For this review, take the finished solid that the model builds, in its own axes (mm). A direction names the side the tool comes from. Round coordinates to 2 decimals unless told otherwise and drop trailing zeros. Write each loop counter-clockwise with the first axis right and the second up, starting at its lowest first coordinate (ties: lowest second). Pieces come first, ordered by that corner, then holes.
from build123d import *

# Parameters (mm, degrees)
F1_DEPTH  = 43
F2_R      = 4
F3_DEPTH  = 6
F4_R      = 1.5
F5_DEPTH  = 25
F4_R_2    = 3
F6_DEPTH  = 1.5
F7_W      = 10
F7_H      = 7
F8_DEPTH  = 5
F10_DEPTH = 50
F11_R     = 2


with BuildPart() as f1:
    # F0 (on Front) → F1 (new body, symmetric)
    with BuildSketch(Plane.XZ):
        with BuildLine():
            Line((0, 11.5), (0, 67))
            Line((0, 67), (-3, 67))
            Line((-3, 67), (-3, 0))
            Line((-3, 0), (23, 0))
            Line((23, 0), (23, 13))
            Line((23, 13), (20, 13))
            Line((20, 13), (18, 11))
            Line((18, 11), (0.5, 11))
            ThreePointArc((0.5, 11), (0.146447, 11.146447), (0, 11.5))
        make_face()
    extrude(amount=F1_DEPTH, both=True)

    # F2 (on face) → F3 (cut)
    with BuildSketch(Plane(origin=(0, 0, 0), x_dir=(1, 0, 0), z_dir=(0, 0, -1))):
        with Locations((3, -33)):
            Circle(F2_R)
        with Locations((3, -8)):
            Circle(F2_R)
        with Locations((3, 32)):
            Circle(F2_R)
    extrude(amount=-F3_DEPTH, mode=Mode.SUBTRACT)

    # F4 (on face) → F5 (cut)
    with BuildSketch(Plane.XY.offset(11)):
        with Locations((3, 33)):
            Circle(F4_R)
        with Locations((3, 8)):
            Circle(F4_R)
        with Locations((3, -32)):
            Circle(F4_R)
    extrude(amount=-F5_DEPTH, mode=Mode.SUBTRACT)

    # F4 (on face) → F6 (cut, symmetric)
    with BuildSketch(Plane.XY.offset(11)):
        with Locations((3, 8)):
            Circle(F4_R_2)
        with Locations((3, 8)):
            Circle(F4_R, mode=Mode.SUBTRACT)
        with Locations((3, 33)):
            Circle(F4_R_2)
        with Locations((3, 33)):
            Circle(F4_R, mode=Mode.SUBTRACT)
        with Locations((3, -32)):
            Circle(F4_R_2)
        with Locations((3, -32)):
            Circle(F4_R, mode=Mode.SUBTRACT)
    extrude(amount=F6_DEPTH, both=True, mode=Mode.SUBTRACT)

    # F7 (on face) → F8 (join)
    with BuildSketch(Plane.XY.offset(11)):
        with Locations((10, 39.5)):
            Rectangle(F7_W, F7_H)
        with Locations((10, -19.5)):
            Rectangle(F7_W, F7_H)
    extrude(amount=F8_DEPTH)

    # F9 (on Front) → F10 (cut, symmetric)
    with BuildSketch(Plane.XZ):
        Polygon((5, 19), (5, 11), (13, 19), align=None)
    extrude(amount=F10_DEPTH, both=True, mode=Mode.SUBTRACT)

    # F11
    f11_edges = [f1.edges().sort_by_distance(p)[0] for p in [
        (23, -43, 6.5),
        (23, 43, 6.5),
        (-1.5, -43, 67),
        (-1.5, 43, 67),
    ]]
    fillet(f11_edges, radius=F11_R)


solid = f1.part
(1) We need section C-C, the plane z = 57. Give the boundary of the cut face in (x, y).
Geometry check:
outline: (-3, -43) - (0, -43) - (0, 43) - (-3, 43) - close
(2) We need section B-B, the plane x = 3. State how many separate pieces and enclosed holes the cut face has, and give its area (4 significant figures).
Geometry check:
separate pieces: 4
enclosed holes: 0
area: 743.5 mm2
(3) Mouldability with a two-part tool opening along Y and no side actions: class faces 5 (the face through (23, -1, 6)), 6 (the face through (11, 36, 13)), 7 (the face through (9, 43, 13)) as pulls with the +Y half, pulls with the -Y half, needs draft (parallel to the pull), parting line crosses it, or undercut.
Geometry check:
face 5: needs draft
face 6: undercut
face 7: pulls with the +Y half
(4) For pin 1 Ø3.5 at (x, y) = (3, 33) entering from -Z; pin 2 Ø12 at (x, y) = (9.5, -17) entering from +Z; pin 3 Ø1.5 at (x, y) = (21.5, 13.5) entering from +Z, all flat-tipped, find the tip position at first contact; note any pin that passes through.
Geometry check:
pin 1: stops at z = 6
pin 2: stops at z = 16
pin 3: stops at z = 13
(5) For faces 1 (the face through (5, 8, 6)), 2 (the face through (11, -16, 13)), 3 (the face through (19, -1, 12)), 4 (the face through (22, -1, 13)), list the 3-axis set-ups (+Z, -Z, +X, -X, +Y, -Y) from which the entire face can be reached by the end or side of a thin tool; tool diameter is ignored.
Geometry check:
face 1: -Z
face 2: +Z
face 3: +Z, +Y, -Y
face 4: +Z, +X, +Y, -Y
(6) For line 1 along Y through (x, z) = (3, 10.35); line 2 along Y through (x, z) = (3, 7.75); line 3 along X through (y, z) = (8, 3.1), list the stretches that pass through material, from the lowest coordinate up.
Geometry check:
line 1: y = -43 to -35, -29 to 5, 11 to 30, 36 to 43
line 2: y = -43 to -33.5, -30.5 to 6.5, 9.5 to 31.5, 34.5 to 43
line 3: x = -3 to -1, 7 to 23
(7) We need section A-A, the plane y = 23.5. Give the boundary of the cut face in (x, z), and give its area (3 significant figures).
Geometry check:
outline: (-3, 0) - (23, 0) - (23, 13) - (20, 13) - (18, 11) - (0.5, 11) arc R0.5 cw to (0, 11.5) - (0, 67) - (-3, 67) - close
area: 462 mm2
